The model under review builds one solid part; all positions refer to its coordinate system, in mm. Face numbers are marked on the shaded views. Coordinates: 2 decimals unless noted, no trailing zeros. Write each loop counter-clockwise with the first axis right and the second up, starting at its lowest first coordinate (ties: lowest second). Pieces come first, ordered by that corner, then holes.
1) Mouldability with a two-part tool opening along X and no side actions: class the marked faces 1, 2 and 3 as released by +X, released by -X, zero draft, split by the parting line, or undercut.
2) Add section C-C, the plane y = 283. State the section outline as (x, z) points, then the cut area to 3 significant figures.
3) Add section A-A, the plane z = 5.5. State the section outline as (x, y) points.
4) Add section B-B, the plane x = -63.5. State the section outline as (y, z) points, then the cut area to 3 significant figures.
5) For line 1 (X direction, y = 153, z = 2.75); line 2 (X direction, y = 190, z = 1.5); line 3 (Y direction, x = 30, z = 2), list the stretches that pass through material, from the lowest coordinate up.
6) For P1, Ø2, axis at x = 28.5, z = 4, coming from the -Y side; P2, Ø1.5, axis at y = 121, z = 9, coming from the +X side; P3, Ø1, axis at y = 287, z = 6, coming from the +X side, all flat-tipped, find the tip position at first contact; note any pin that passes through.
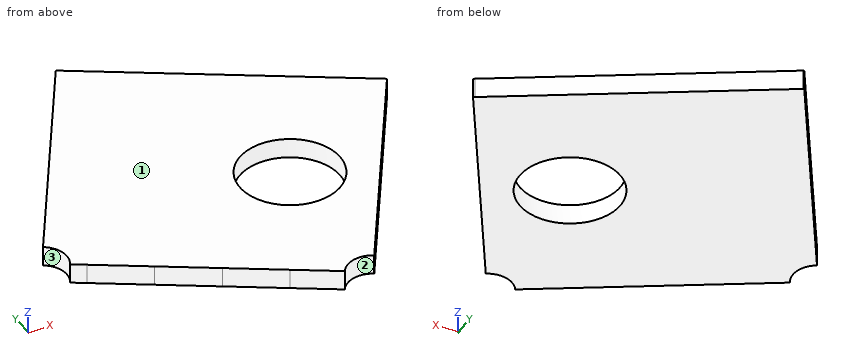
Autodesk Inventor part; units mm, degrees
ref_plane "YZ Plane" through (0, 0, 0) normal (1, 0, 0) x (0, 1, 0)
ref_plane "XZ Plane" through (0, 0, 0) normal (0, 1, 0) x (-1, 0, 0)
ref_plane "XY Plane" through (0, 0, 0) normal (0, 0, 1) x (1, 0, 0)
ref_plane "Work Plane1" through (0, 0, 0) normal (0, 0, 1) x (1, 0, 0)
sketch "Sketch1" plane through (0, 0, 0) normal (0, 0, 1) x (1, 0, 0)
  circle A0 centre (68.259454, 214.654052) radius 4
  line L0 (64.259454, -185.345948) -> (64.259454, -225.345948)
  arc A1 (72.259454, -185.345948) -> (64.259454, -185.345948) centre (68.259454, -185.345948) ccw
  line L1 (72.259454, -225.345948) -> (72.259454, -185.345948)
  arc A2 (64.259454, -225.345948) -> (72.259454, -225.345948) centre (68.259454, -225.345948) ccw
  line L2 (-101.259454, 230.542101) -> (-90.867149, 224.542101)
  line L3 (-90.867149, 224.542101) -> (-108.867149, 193.365186)
  line L4 (-108.867149, 193.365186) -> (-119.259454, 199.365186)
  line L5 (-137.259454, 168.188271) -> (-119.259454, 199.365186)
  line L6 (-137.259454, 168.188271) -> (-106.082539, 150.188271)
  line L7 (-106.082539, 150.188271) -> (-112.082539, 139.795967)
  line L8 (-80.905625, 121.795967) -> (-112.082539, 139.795967)
  line L9 (-80.905625, 121.795967) -> (-74.905625, 132.188271)
  line L10 (-74.905625, 132.188271) -> (-43.72871, 114.188271)
  line L11 (-43.72871, 114.188271) -> (-49.72871, 103.795967)
  line L12 (-18.551796, 85.795967) -> (-49.72871, 103.795967)
  line L13 (-18.551796, 85.795967) -> (-12.551796, 96.188271)
  line L14 (-12.551796, 96.188271) -> (18.625119, 78.188271)
  line L15 (18.625119, 78.188271) -> (12.625119, 67.795967)
  line L16 (23.259454, 61.656231) -> (12.625119, 67.795967)
  line L17 (23.259454, -7.001047) -> (23.259454, 61.656231)
  line L18 (23.259454, -7.001047) -> (35.259454, -7.001047)
  line L19 (35.259454, -7.001047) -> (35.259454, -43.001047)
  line L20 (35.259454, -43.001047) -> (23.259454, -43.001047)
  line L21 (23.259454, -79.001047) -> (23.259454, -43.001047)
  line L22 (23.259454, -79.001047) -> (35.259454, -79.001047)
  line L23 (35.259454, -79.001047) -> (35.259454, -115.001047)
  line L24 (35.259454, -115.001047) -> (23.259454, -115.001047)
  line L25 (23.259454, -151.001047) -> (23.259454, -115.001047)
  line L26 (23.259454, -151.001047) -> (35.259454, -151.001047)
  line L27 (35.259454, -151.001047) -> (35.259454, -187.001047)
  line L28 (35.259454, -187.001047) -> (23.259454, -187.001047)
  line L29 (23.259454, -223.001047) -> (23.259454, -187.001047)
  line L30 (23.259454, -223.001047) -> (35.259454, -223.001047)
  line L31 (35.259454, -223.001047) -> (35.259454, -259.001047)
  line L32 (35.259454, -259.001047) -> (23.259454, -259.001047)
  line L33 (23.259454, -295.001047) -> (23.259454, -259.001047)
  line L34 (23.259454, -295.001047) -> (35.259454, -295.001047)
  line L35 (35.259454, -295.001047) -> (35.259454, -331.001047)
  line L36 (105.759454, -290.297853) -> (35.259454, -331.001047)
  arc A3 (105.759454, -290.297853) -> (143.259454, -225.345948) centre (68.259454, -225.345948) ccw
  line L37 (143.259454, -185.345948) -> (143.259454, -225.345948)
  arc A4 (143.259454, -185.345948) -> (125.301159, -136.650529) centre (68.259454, -185.345948) ccw
  arc A5 (114.658634, -107.792431) -> (125.301159, -136.650529) centre (159.105469, -107.792431) ccw
  line L38 (114.658634, 129.266291) -> (114.658634, -107.792431)
  arc A6 (128.128133, 169.479488) -> (114.658634, 129.266291) centre (181.421641, 129.266291) ccw
  arc A7 (128.128133, 169.479488) -> (62.965391, 289.466971) centre (68.259454, 214.654052) ccw
  arc A8 (5.90664, 302.61499) -> (62.965391, 289.466971) centre (55.90664, 389.21753) ccw
  line L39 (-43.259454, 331.001047) -> (5.90664, 302.61499)
  line L40 (-65.259454, 292.89593) -> (-43.259454, 331.001047)
  line L41 (-65.259454, 292.89593) -> (-54.867149, 286.89593)
  line L42 (-54.867149, 286.89593) -> (-72.867149, 255.719015)
  line L43 (-72.867149, 255.719015) -> (-83.259454, 261.719015)
  line L44 (-101.259454, 230.542101) -> (-83.259454, 261.719015)
  circle A9 centre (28.259454, 174.654052) radius 30
  line L45 (71.945627, 130.542101) -> (61.553322, 136.542101)
  line L46 (61.553322, 136.542101) -> (79.553322, 167.719015)
  line L47 (79.553322, 167.719015) -> (89.945627, 161.719015)
  line L48 (89.945627, 161.719015) -> (71.945627, 130.542101)
  line L49 (-32.867149, 325.001047) -> (-54.867149, 286.89593)
  line L50 (61.553322, 136.542101) -> (30.062941, 81.999161)
  line L51 (-12.551796, 96.188271) -> (18.625119, 78.188271)
  line L52 (-38.001123, 314.108743) -> (112.687297, 227.108743)
  line L53 (-54.867149, 286.89593) -> (-72.867149, 255.719015)
  line L54 (-74.905625, 132.188271) -> (-43.72871, 114.188271)
  line L55 (-38.001123, 314.108743) -> (112.687297, 227.108743)
  line L56 (119.553322, 237.001047) -> (79.553322, 167.719015)
  line L57 (-38.867149, 314.608743) -> (-126.867149, 162.188271)
  line L58 (-126.867149, 162.188271) -> (25.553322, 74.188271)
  line L59 (25.553322, 74.188271) -> (113.553322, 226.608743)
  line L60 (113.553322, 226.608743) -> (-38.867149, 314.608743)
  circle A10 centre (-126.867149, 162.188271) radius 15
  circle A11 centre (25.553322, 74.188271) radius 15
  circle A12 centre (28.259454, 174.654052) radius 30
  point P0 (0, 0)
  point P1 (37.343087, 270.608743)
  point P2 (37.343087, 270.608743)
  point P3 (70.553322, 152.130558)
  point P4 (-59.317167, 123.188271)
  point P5 (12.562941, 81.688271)
  point P6 (33.053322, 87.178653)
  point P7 (-119.367149, 175.178653)
  point P8 (-113.876768, 154.688271)
  dimension "d0" = 30
  dimension "d1" = 30
  dimension "d2" = 60
extrude "Extrusion1" add sketch "Sketch1" along normal blind 12 contours A0 | L57 L42 L49 L60 L52 L56 L46 L50 A11 L14 L58 L10 L6 A10 L3
move faces "Move1" translate (-0.5, -0.866025, 0) faces at (62.457823, 256.108743, 4)
sketch "Sketch2" plane through (0, 0, 12) normal (0, 0, 1) x (1, 0, 0)
  line L0 (-39.367149, 313.742717) -> (-119.367149, 175.178653)
  arc A0 (-113.876768, 154.688271) -> (-119.367149, 175.178653) centre (-126.867149, 162.188271) ccw
  line L1 (-113.876768, 154.688271) -> (12.562941, 81.688271)
  arc A1 (33.053322, 87.178653) -> (12.562941, 81.688271) centre (25.553322, 74.188271) ccw
  line L2 (33.053322, 87.178653) -> (113.053322, 225.742717)
  line L3 (113.053322, 225.742717) -> (-39.367149, 313.742717)
  circle A2 centre (28.259454, 174.654052) radius 30
  point P0 (0, 0)
equation "\"d1\" = d0"
properties part number "wooden_internal"
Geometry results:
1. face 1: zero draft
1. face 2: undercut
1. face 3: released by -X
2. outline: (-57.12, 0) - (13.88, 0) - (13.88, 12) - (-57.12, 12) - close
2. area: 852 mm2
3. outline: (-119.37, 175.18) arc R15 cw to (-113.88, 154.69) - (12.56, 81.69) arc R15 cw to (33.05, 87.18) - (113.05, 225.74) - (-39.37, 313.74) - close; hole circle Ø60 at (28.26, 174.65)
4. outline: (125.6, 0) - (271.94, 0) - (271.94, 12) - (125.6, 12) - close
4. area: 1,760 mm2
5. line 1: x = -110.95 to 7.5, 49.02 to 71.06
5. line 2: x = -110.81 to 2.48, 54.04 to 92.42
5. line 3: y = 88.51 to 144.7, 204.6 to 273.69
6. P1: stops at y = 88.66
6. P2: stops at x = 53.01
6. P3: stops at x = 7.82
